Verification items for this drawing (mm, ordinates from the low corner). Coordinates: 2 decimals unless noted, no trailing zeros. Loops run counter-clockwise (first coordinate to the right, second up) from the corner with the lowest first, then second, coordinate; pieces in that order, holes last. Notation, with made-up numbers: (35.5, -21) - (66.5, -21) arc R30 cw to (66.5, 8) - close; hole circle Ø3 at (-24, 48.5). An arc over 180 degrees is marked (long way). One line per item, written item: value. Start each with the question number.
(1) Section check A-A (x = 150). Record the boundary of the cut face in (y, z).
(2) Section check C-C (y = 55). Record the boundary of the cut face in (x, z).
(3) Gauge pin test, flat ends, axial feed: P1, Ø6, axis at x = 123.48, y = 33.48, coming from the +Z side; P2, Ø3.5, axis at x = 207, z = 3, coming from the +Y side. Record the tip position at first contact, or that the pin passes through.
(4) Section check B-B (y = 8.5). Record the boundary of the cut face in (x, z), plus the area to 3 significant figures.
(5) Section check D-D (x = 3). Record the boundary of the cut face in (y, z), plus the area to 3 significant figures.
(6) Thickness scan on probe 1 along Y at (x, z) = (13, 3.2); probe 2 along X at (y, z) = (8.75, 3); probe 3 along X at (y, z) = (32.5, 3.7) (1 decimal). Record the ranges inside material, lowest first. Write a range as [from, to].
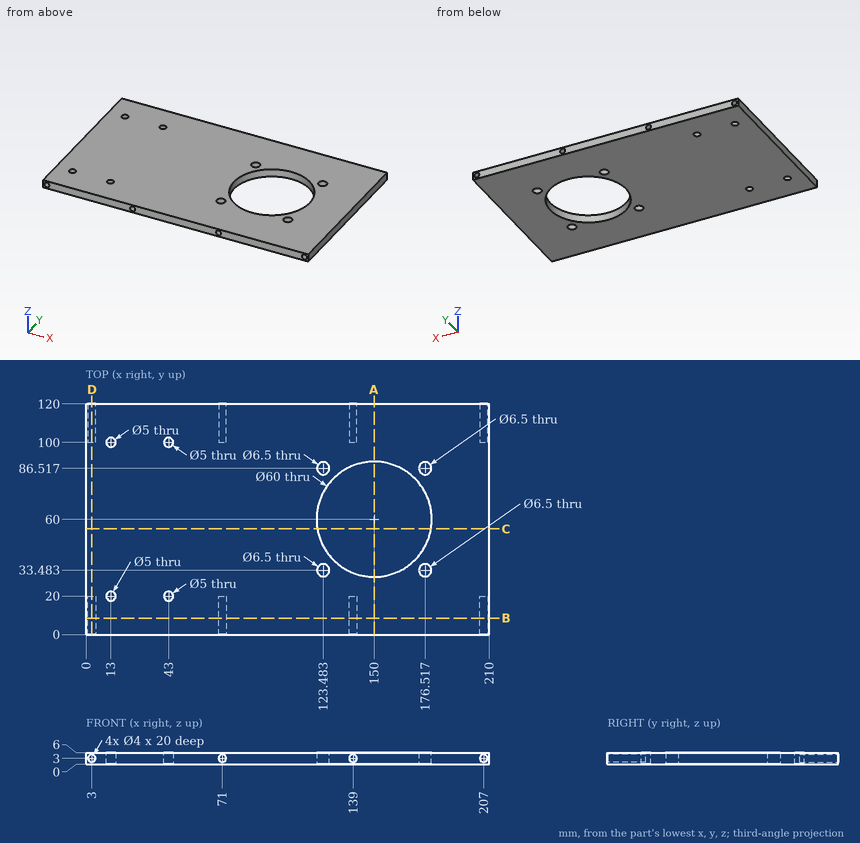
Responses:
1. outline: (0, 0) - (30, 0) - (30, 6) - (0, 6) - close; (90, 0) - (120, 0) - (120, 6) - (90, 6) - close
2. outline: (0, 0) - (120.42, 0) - (120.42, 6) - (0, 6) - close; (179.58, 0) - (210, 0) - (210, 6) - (179.58, 6) - close
3. P1: passes through
3. P2: stops at y = 100
4. outline: (0, 0) - (210, 0) - (210, 6) - (0, 6) - close; hole circle Ø4 at (3, 3); hole circle Ø4 at (71, 3); hole circle Ø4 at (139, 3); hole circle Ø4 at (207, 3)
4. area: 1,210 mm²
5. outline: (0, 0) - (120, 0) - (120, 1) - (100, 1) - (100, 5) - (120, 5) - (120, 6) - (0, 6) - (0, 5) - (20, 5) - (20, 1) - (0, 1) - close
5. area: 560 mm²
6. probe 1: y = [0, 17.5], [22.5, 97.5], [102.5, 120]
6. probe 2: x = [0, 1], [5, 69], [73, 137], [141, 205], [209, 210]
6. probe 3: x = [0, 120.4], [126.6, 138], [162, 173.4], [179.6, 210]
